Build history of the part. All positions in model axes, mm. A direction names the side the tool comes from. Give positions to 0.01 mm unless a question says otherwise; leave off trailing zeros. Loops run counter-clockwise (first coordinate to the right, second up) from the corner with the lowest first, then second, coordinate; pieces in that order, holes last. Notation, with made-up numbers: M 43.25,6.5 L 77.25,6.5 A21 ccw 77.25,30.5 Z; hole C 4.5,15.25 d10. An arc over 180 degrees is marked long. Answer in a Markdown table with one row per item. Add a question column.
```python
from build123d import *

# Parameters (mm, degrees)
SKETCH1_R           = 1.8288
BOSS_EXTRUDE1_DEPTH = 3.175
FILLET1_R           = 3.175


with BuildPart() as part:
    # Sketch1 → Boss-Extrude1 (new body)
    # profile 1 of 3: a face of its own
    with BuildSketch(Plane(origin=(0, 0, 0), x_dir=(0, 0, -1), z_dir=(1, 0, 0))):
        with BuildLine():
            Line((-19.639409497, -3.81), (19.639409497, -3.81))
            Line((19.639409497, -3.81), (4.259709497, 26.9494))
            ThreePointArc((4.259709497, 26.9494), (0, 22.689690503), (-4.259709497, 26.9494))
            Line((-4.259709497, 26.9494), (-19.639409497, -3.81))
        make_face()
        with Locations((-13.4747, 0)):
            Circle(SKETCH1_R, mode=Mode.SUBTRACT)
        with Locations((13.4747, 0)):
            Circle(SKETCH1_R, mode=Mode.SUBTRACT)
    # profile 2 of 3: a face of its own
    with BuildSketch(Plane(origin=(0, 0, 0), x_dir=(0, 0, -1), z_dir=(1, 0, 0))):
        with BuildLine():
            ThreePointArc((-4.259709497, 26.9494), (0, 22.689690503), (4.259709497, 26.9494))
            Line((4.259709497, 26.9494), (0, 35.468818994))
            Line((0, 35.468818994), (-4.259709497, 26.9494))
        make_face()
        with Locations((0, 26.9494)):
            Circle(SKETCH1_R, mode=Mode.SUBTRACT)
    # profile 3 of 3: a face of its own
    with BuildSketch(Plane(origin=(0, 0, 0), x_dir=(0, 0, -1), z_dir=(1, 0, 0))):
        with BuildLine():
            Line((0, 35.468818994), (4.259709497, 26.9494))
            Line((4.259709497, 26.9494), (4.259709497, 126.9494))
            ThreePointArc((4.259709497, 126.9494), (0, 131.209109497), (-4.259709497, 126.9494))
            Line((-4.259709497, 126.9494), (-4.259709497, 26.9494))
            Line((-4.259709497, 26.9494), (0, 35.468818994))
        make_face()
        with Locations((0, 126.9494)):
            Circle(SKETCH1_R, mode=Mode.SUBTRACT)
    extrude(amount=BOSS_EXTRUDE1_DEPTH)

    # Fillet1
    fillet1_edges = [part.edges().sort_by_distance(p)[0] for p in [
        (1.5875, -3.81, -19.639409497),
        (1.5875, -3.81, 19.639409497),
        (1.5875, 26.9494, 4.259709497),
        (1.5875, 26.9494, -4.259709497),
    ]]
    fillet(fillet1_edges, radius=FILLET1_R)


solid = part.part
```
(1) Slice it at B-B, the plane x = 1.1. State how many separate pieces and enclosed holes the cut face has, then the cut area to 3 significant figures.
(2) Slice it at D-D, the plane z = 7. Give the cut face in (x, y) (3 decimals).
(3) Tool access for faces 4 (the cylindrical face through (1.565, 28.763, 0.238)), 5 (the flat face through (2, 77, -4.26)): list every direction of +Z, -Z, +X, -X, +Y, -Y with a clear straight run to the whole face (end or side of a thin tool).
(4) Slice it at A-A, the plane z = 0. Give the cut face in (x, y) (3 decimals), then the cut area to 3 significant figures.
(5) Pull direction Y, two halves, no side cores. Call faces 1 (the cylindrical face through (1.61, -2.266, -17.226)), 2 (the cylindrical face through (1.57, -1.11, -12.02)), 3 (the flat face through (2, 78, 4.26)): +Y half, -Y half, draft (parallel to the pull), parting line (faces both ways), or undercut.
(6) Slice it at C-C, the plane y = 101. Give the cut face in (x, z) (3 decimals), then the cut area to 3 significant figures.
(7) Wall check: line 1 (Y direction, x = 2.1, z = 0); line 2 (Z direction, x = 0.7, y = 64); line 3 (Y direction, x = 0.7, z = 1.5). Give the ranges that are in metal, low to high.
Solution:
| question | item | result |
|---|---|---|
| 1 | separate pieces | 1 |
| 1 | enclosed holes | 4 |
| 1 | area | 1,560 mm^2 |
| 2 | outline | M 0,-3.81 L 3.175,-3.81 L 3.175,21.469 L 0,21.469 Z |
| 3 | face 4 | +X, -X |
| 3 | face 5 | -Z, +X, -X, +Y |
| 4 | outline | M 0,-3.81 L 3.175,-3.81 L 3.175,25.121 L 0,25.121 Z; M 0,28.778 L 3.175,28.778 L 3.175,125.121 L 0,125.121 Z; M 0,128.778 L 3.175,128.778 L 3.175,131.209 L 0,131.209 Z |
| 4 | area | 405 mm^2 |
| 5 | face 1 | parting line |
| 5 | face 2 | undercut |
| 5 | face 3 | draft |
| 6 | outline | M 0,-4.26 L 3.175,-4.26 L 3.175,4.26 L 0,4.26 Z |
| 6 | area | 27.0 mm^2 |
| 7 | line 1 | -3.81 to 25.12, 28.78 to 125.12, 128.78 to 131.21 |
| 7 | line 2 | -4.26 to 4.26 |
| 7 | line 3 | -3.81 to 25.9, 28 to 125.9, 128 to 130.94 |
